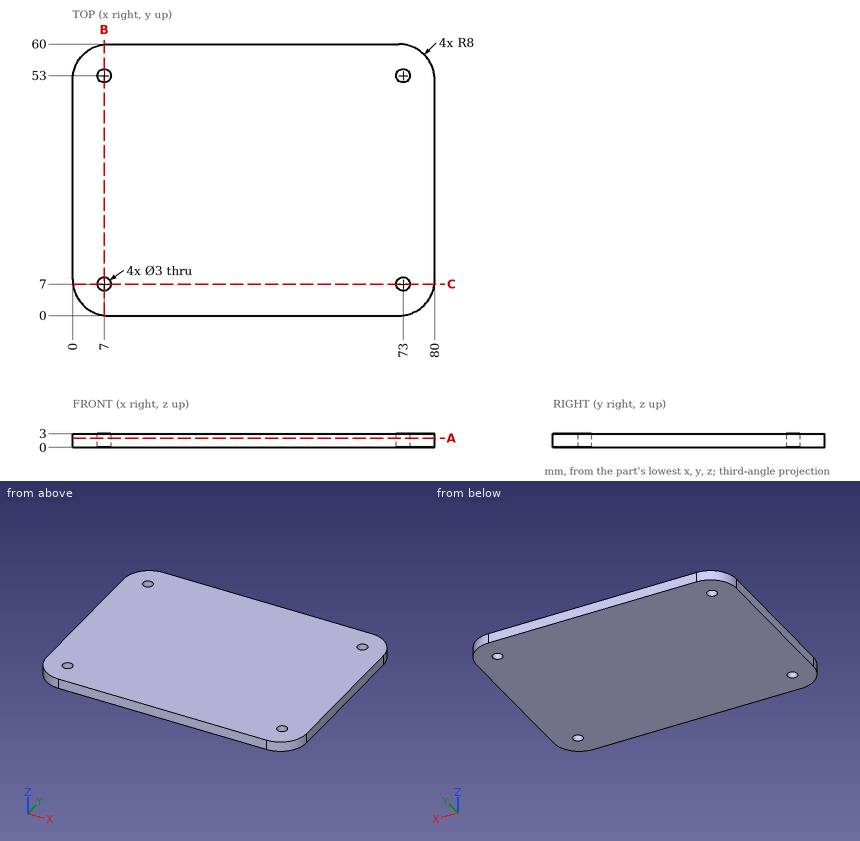
The drawing under review shows one solid part. Ordinate dimensions are in mm from its lowest x, y, z. Round coordinates to 2 decimals unless told otherwise and drop trailing zeros. Order: outer loops, then holes, each group sorted by start corner. A loop starts at its lowest first (then second) coordinate and runs counter-clockwise, first axis right, second up. Notation, with made-up numbers: (69, 62) - (113, 62) arc R23 ccw to (113, 95) - close; hole circle Ø8 at (72.5, 78). An arc over 180 degrees is marked (long way). Return JSON: item names as keys, results as strings.
Q1. For pin 1 Ø1 at (y, z) = (6, 0.5) entering from +X, flat-tipped, find the tip position at first contact; note if it passes through.
Computed values:
{"pin 1": "stops at x = 79.86"}
Q2. Consider section B-B on x = 7. Write out the cut boundary in (y, z).
Computed values:
{"outline": "(0.06, 0) - (5.5, 0) - (5.5, 3) - (0.06, 3) - close; (8.5, 0) - (51.5, 0) - (51.5, 3) - (8.5, 3) - close; (54.5, 0) - (59.94, 0) - (59.94, 3) - (54.5, 3) - close"}
Q3. Wall thickness on L1, parallel to Y at x = 7, z = 1.9; L2, parallel to Y at x = 72, z = 2.85; L3, parallel to X at y = 6.5, z = 0.2: over which ranges is each line inside the solid? List them lowest first. Write a range as [from, to].
Computed values:
{"L1": "y = [0.06, 5.5], [8.5, 51.5], [54.5, 59.94]", "L2": "y = [0, 5.88], [8.12, 51.88], [54.12, 60]", "L3": "x = [0.14, 5.59], [8.41, 71.59], [74.41, 79.86]"}
Q4. Consider section A-A on z = 2. Write out the cut boundary in (x, y).
Computed values:
{"outline": "(0, 8) arc R8 ccw to (8, 0) - (72, 0) arc R8 ccw to (80, 8) - (80, 52) arc R8 ccw to (72, 60) - (8, 60) arc R8 ccw to (0, 52) - close; hole circle Ø3 at (7, 7); hole circle Ø3 at (7, 53); hole circle Ø3 at (73, 7); hole circle Ø3 at (73, 53)"}
Q5. Consider section C-C on y = 7. Write out the cut boundary in (x, z), plus the area to 3 significant figures.
Computed values:
{"outline": "(0.06, 0) - (5.5, 0) - (5.5, 3) - (0.06, 3) - close; (8.5, 0) - (71.5, 0) - (71.5, 3) - (8.5, 3) - close; (74.5, 0) - (79.94, 0) - (79.94, 3) - (74.5, 3) - close", "area": "222 mm2"}
